Could you check a few things on this model? Use its own coordinates, in mm. Face numbers are marked on the shaded views. A direction names the side the tool comes from. Round coordinates to 2 decimals unless told otherwise and drop trailing zeros. Order: outer loops, then holes, each group sorted by start corner. A loop starts at its lowest first (then second) coordinate and runs counter-clockwise, first axis right, second up.
```python
from build123d import *

# Parameters (mm, degrees)
F0_W          = 38
F0_H          = 38
F0_W_2        = 34
F0_H_2        = 34
F1_DEPTH      = 8
F3_DEPTH      = 1
F5_DEPTH      = 8
F6_R          = 0.75
F7_DEPTH      = 50.7
F7_DEPTH_BACK = 53.4
F8_R          = 5


with BuildPart() as f1:
    # F0 (on Top) → F1 (new body)
    with BuildSketch(Plane.XY):
        with Locations((19, 19)):
            Rectangle(F0_W, F0_H)
        with Locations((19, 19)):
            Rectangle(F0_W_2, F0_H_2, mode=Mode.SUBTRACT)
    extrude(amount=F1_DEPTH)

    # F2 (on face) → F3 (cut)
    with BuildSketch(Plane.XY.offset(8)):
        Polygon((13, 0), (19, 0), (25, 0), (25, 1), (19, 1), (13, 1), align=None)
    extrude(amount=-F3_DEPTH, mode=Mode.SUBTRACT)

    # F4 (on face) → F5 (join)
    with BuildSketch(Plane.XY.offset(8)):
        Polygon((0, 38), (0, 0), (2, 0), (2, 2), (2, 36), (2, 38), align=None)
        Polygon((38, 38), (36, 38), (36, 36), (36, 2), (36, 0), (38, 0), align=None)
    extrude(amount=F5_DEPTH)

    # F6 (on face) → F7 (cut, two sides)
    with BuildSketch(Plane(origin=(36, 0, 0), x_dir=(0, -1, 0), z_dir=(-1, 0, 0))) as f7_sk:
        with Locations((-31.5038709193, 12)):
            Circle(F6_R)
        with Locations((-12.9723072276, 12)):
            Circle(F6_R)
    extrude(amount=-F7_DEPTH, mode=Mode.SUBTRACT)
    extrude(f7_sk.sketch, amount=F7_DEPTH_BACK, mode=Mode.SUBTRACT)

    # F8
    f8_edges = [f1.edges().sort_by_distance(p)[0] for p in [
        (1, 0, 16),
        (37, 0, 16),
        (37, 38, 16),
        (1, 38, 16),
    ]]
    fillet(f8_edges, radius=F8_R)


solid = f1.part
```
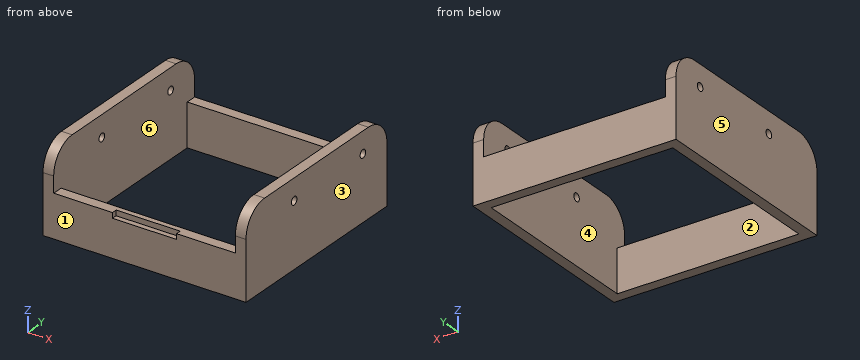
Q1. Imagine slicing it at B-B, the plane z = 5.5. Please give me the cut outline in (x, y), then the cut area to 3 significant figures.
Q2. For the marked faces 1 and 2, which set-ups out of +Z, -Z, +X, -X, +Y, -Y let a thin tool reach every point of the face, with its end or its side?
Q3. Imagine slicing it at D-D, the plane z = 14.5. Please give me the cut outline in (x, y).
Q4. For P1, Ø2, axis at x = 14.5, y = 36.5, coming from the +Z side; P2, Ø0.5, axis at x = 16, y = 0.5, coming from the +Z side; P3, Ø0.5, axis at x = 18, z = 7.5, coming from the -Y side, each with a flat end and sliding along its axis, tell me the tip position at first contact or that it passes through.
Q5. We'd pull the mould along X, two halves only. Please class the marked faces 3, 4, 5 and 6: released by +X, released by -X, zero draft, split by the parting line, or undercut.
Q6. Imagine slicing it at C-C, the plane y = 11.5. Please give me the cut outline in (x, z).
Q7. Imagine slicing it at A-A, the plane x = 14. Please give me the cut outline in (y, z), then the cut area to 3 significant figures.
Q8. I need wall thicknesses on L1, parallel to Y at x = 16.5, z = 4.5; L2, parallel to Y at x = 0.75, z = 12. Which ranges of each line are inside material? Lowest first, please.
Filled in:
1. outline: (0, 0) - (38, 0) - (38, 38) - (0, 38) - close; hole (2, 2) - (36, 2) - (36, 36) - (2, 36) - close
1. area: 288 mm2
2. face 1: +Z, -Z, +X, -X, -Y
2. face 2: +Z, -Z
3. outline: (0, 1.43) - (2, 1.43) - (2, 36.57) - (0, 36.57) - close; (36, 1.43) - (38, 1.43) - (38, 36.57) - (36, 36.57) - close
4. P1: stops at z = 8
4. P2: stops at z = 7
4. P3: stops at y = 1
5. face 3: released by +X
5. face 4: undercut
5. face 5: released by -X
5. face 6: undercut
6. outline: (0, 0) - (2, 0) - (2, 16) - (0, 16) - close; (36, 0) - (38, 0) - (38, 16) - (36, 16) - close
7. outline: (0, 0) - (2, 0) - (2, 8) - (1, 8) - (1, 7) - (0, 7) - close; (36, 0) - (38, 0) - (38, 8) - (36, 8) - close
7. area: 31.0 mm2
8. L1: y = 0 to 2, 36 to 38
8. L2: y = 0.1 to 12.22, 13.72 to 30.75, 32.25 to 37.9
